Design review of the part built by this model. Coordinates are the model's own, in mm. A direction names the side the tool comes from. Coordinates: 2 decimals unless noted, no trailing zeros. Loops run counter-clockwise (first coordinate to the right, second up) from the corner with the lowest first, then second, coordinate; pieces in that order, holes last. Notation, with made-up numbers: (23.5, 28) - (57.5, 28) arc R24 cw to (57.5, 63) - close; hole circle Ø2 at (-24, -35). An arc over 180 degrees is marked (long way). Answer in a Markdown table with one row per item. Add a question column.
(1) For faces 1 (the face through (0, 2, -1.9)), 2 (the face through (1, 1, 0)), 3 (the face through (0, 0, -1.05)), list the 3-axis set-ups (+Z, -Z, +X, -X, +Y, -Y) from which the entire face can be reached by the end or side of a thin tool; tool diameter is ignored.
(2) The part is to be moulded in two halves that separate along Y. For faces 4 (the face through (-0.51, -0.86, -0.52)), 5 (the face through (0, 0, -10)), 6 (the face through (-1.474, -0.065, -5.893)), say which applies: released by +Y, released by -Y, zero draft, split by the parting line, or undercut.
(3) To check wall thickness, follow L1, parallel to Z at x = 2.5, y = 0.25; L2, parallel to Y at x = 0, z = -8.25 (3 decimals); L3, parallel to Z at x = -0.75, y = 0. State the ranges of each line that lie inside material, in increasing order. Write a range as [from, to].
(4) We need section B-B, the plane z = -4.25. Write out the cut boundary in (x, y) (3 decimals).
(5) We need section A-A, the plane y = 0. Write out the cut boundary in (x, z) (3 decimals), plus the area to 3 significant figures.
(6) Clearance check with flat-ended pins moving along their axes: pin 1 (4 mm diameter, centred on x = -1.5, z = -5.5, fed in from -Y) (3 decimals); pin 2 (3 mm diameter, centred on y = 0.5, z = -6.5, fed in from +X) (3 decimals); pin 3 (2 mm diameter, centred on y = -1.5, z = -5.5, fed in from -X). State where each tip first meets the part, or that it passes through.
from build123d import *

# Parameters (mm, degrees)
FILLET1_R          = 1
CUT_EXTRUDE1_DEPTH = 1.05


with BuildPart() as part:
    # Sketch1 → Revolve1 (revolve)
    with BuildSketch(Plane(origin=(0, 0, 0), x_dir=(0, 0, -1), z_dir=(1, 0, 0)), mode=Mode.PRIVATE) as revolve1_sk:
        Polygon((1.9, 1.475), (1.9, 3.5), (0, 3.5), (0, 0), (10, 0), (10, 1.475), align=None)
    revolve(revolve1_sk.sketch.rotate(Axis((0, 0, 0), (0, 0, -1)), 90), axis=Axis((0, 0, 0), (0, 0, -1)))

    # Fillet1
    fillet1_edges = [part.edges().sort_by_distance(p)[0] for p in [
        (-3.5, 0, 0),
    ]]
    fillet(fillet1_edges, radius=FILLET1_R)

    # Sketch2 → Cut-Extrude1 (cut)
    with BuildSketch(Plane.XY):
        Polygon((0, 1.154700538), (-1, 0.577350269), (-1, -0.577350269), (0, -1.154700538), (1, -0.577350269), (1, 0.577350269), align=None)
    extrude(amount=-CUT_EXTRUDE1_DEPTH, mode=Mode.SUBTRACT)


solid = part.part
Responses:
| question | item | result |
|---|---|---|
| 1 | face 1 | -Z |
| 1 | face 2 | +Z, +X, -X, +Y, -Y |
| 1 | face 3 | +Z |
| 2 | face 4 | undercut |
| 2 | face 5 | zero draft |
| 2 | face 6 | split by the parting line |
| 3 | L1 | z = [-1.9, 0] |
| 3 | L2 | y = [-1.475, 1.475] |
| 3 | L3 | z = [-10, -1.05] |
| 4 | outline | circle Ø2.95 at (0, 0) |
| 5 | outline | (-3.5, -1.9) - (-1.475, -1.9) - (-1.475, -10) - (1.475, -10) - (1.475, -1.9) - (3.5, -1.9) - (3.5, -1) arc R1 ccw to (2.5, 0) - (1, 0) - (1, -1.05) - (-1, -1.05) - (-1, 0) - (-2.5, 0) arc R1 ccw to (-3.5, -1) - close |
| 5 | area | 34.7 mm2 |
| 6 | pin 1 | stops at y = -1.475 |
| 6 | pin 2 | stops at x = 1.475 |
| 6 | pin 3 | stops at x = -1.39 |
